```python
from build123d import *

# Parameters (mm, degrees)
BOSS_EXTRUDE1_DEPTH = 1
SKETCH2_W           = 7
SKETCH2_H           = 18
SKETCH2_R           = 2
BOSS_EXTRUDE2_DEPTH = 4


with BuildPart() as part:
    # Sketch1 → Boss-Extrude1 (new body)
    with BuildSketch(Plane(origin=(0, 0, 0), x_dir=(1, 0, 0), z_dir=(0, 1, 0))):
        Polygon((-9, 0), (9, 0), (9, 3), (6, 3), (6, 14), (9, 14), (9, 18), (-9, 18), (-9, 14), (-6, 14), (-6, 3), (-9, 3), align=None)
    extrude(amount=BOSS_EXTRUDE1_DEPTH)

    # Sketch2 → Boss-Extrude2 (add)
    # profile 1 of 2: a face of its own
    with BuildSketch(Plane(origin=(0, 1, 0), x_dir=(1, 0, 0), z_dir=(0, 1, 0))):
        with Locations((-12.5, 9)):
            Rectangle(SKETCH2_W, SKETCH2_H)
        with Locations(Location((-12.5, 9, 0), (0, 0, 270))):
            Circle(SKETCH2_R, mode=Mode.SUBTRACT)
    # profile 2 of 2: a face of its own
    with BuildSketch(Plane(origin=(0, 1, 0), x_dir=(1, 0, 0), z_dir=(0, 1, 0))):
        with Locations((12.5, 9)):
            Rectangle(SKETCH2_W, SKETCH2_H)
        with Locations(Location((12.5, 9, 0), (0, 0, 90))):
            Circle(SKETCH2_R, mode=Mode.SUBTRACT)
    extrude(amount=-BOSS_EXTRUDE2_DEPTH)


solid = part.part
```
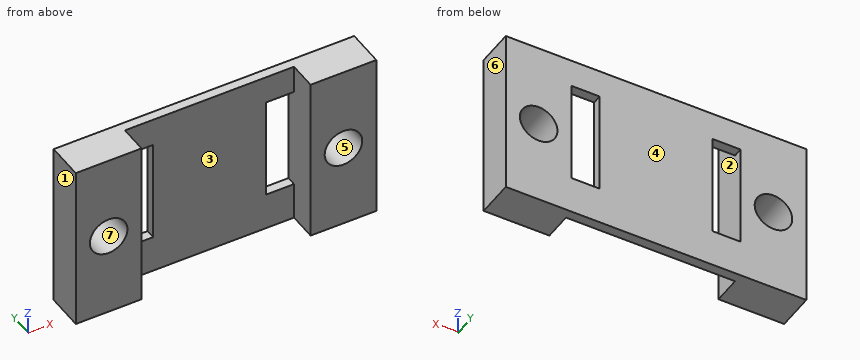
Check sheet for the modelled part. Datum: model origin and axes. Units: mm. Face numbers are marked on the shaded views. A direction names the side the tool comes from. Coordinates: 2 decimals unless noted, no trailing zeros. Write each loop counter-clockwise with the first axis right and the second up, starting at its lowest first coordinate (ties: lowest second). Pieces come first, ordered by that corner, then holes. Notation, with made-up numbers: (56.25, -26) - (66.25, -26) arc R21 ccw to (66.25, -1) - close; hole circle Ø7 at (22, 25). An arc over 180 degrees is marked (long way). One line per question, with ' | ' between items.
Item 1: Thickness scan on line 1 (X direction, y = -1.7, z = -9); line 2 (X direction, y = 0.5, z = -13.25); line 3 (Z direction, x = 12.5, y = -0.7). Record the ranges inside material, lowest first. Write a range as [from, to].
Determined:
line 1: x = [-16, -14.5], [-10.5, -9], [9, 10.5], [14.5, 16] | line 2: x = [-16, -9], [-6, 6], [9, 16] | line 3: z = [-18, -11], [-7, 0]
Item 2: Mould release check, pull along X, two halves, no side actions. Record for the marked faces 4, 5, 6 and 7: pulls with the +X half, pulls with the -X half, needs draft (parallel to the pull), parting line crosses it, or undercut.
Determined:
face 4: needs draft | face 5: undercut | face 6: pulls with the +X half | face 7: undercut
Item 3: Sectioned sample at A-A on y = -1.8. Record the boundary of the cut face in (x, z).
Determined:
outline: (-16, -18) - (-9, -18) - (-9, 0) - (-16, 0) - close; (9, -18) - (16, -18) - (16, 0) - (9, 0) - close; hole circle Ø4 at (-12.5, -9); hole circle Ø4 at (12.5, -9)
Item 4: Gauge pin test, flat ends, axial feed: P1, Ø1.5, axis at x = 3.5, y = -2.5, coming from the -Z side; P2, Ø2, axis at x = -3, z = -3.5, coming from the -Y side. Record the tip position at first contact, or that the pin passes through.
Determined:
P1: passes through | P2: stops at y = 0
Item 5: Access from +Z, -Z, +X, -X, +Y, -Y to the whole of each face (thin tool, end or side, straight path). Record for the marked faces 1, 2 and 3.
Determined:
face 1: +Z, -Z, -X, +Y, -Y | face 2: -Y | face 3: +Z, -Z, -Y
Item 6: Sectioned sample at C-C on z = -9. Record the boundary of the cut face in (x, y), plus the area to 3 significant figures.
Determined:
outline: (-16, -3) - (-14.5, -3) - (-14.5, 1) - (-16, 1) - close; (-10.5, -3) - (-9, -3) - (-9, 1) - (-10.5, 1) - close; (-6, 0) - (6, 0) - (6, 1) - (-6, 1) - close; (9, -3) - (10.5, -3) - (10.5, 1) - (9, 1) - close; (14.5, -3) - (16, -3) - (16, 1) - (14.5, 1) - close | area: 36.0 mm2
Item 7: Sectioned sample at B-B on x = -12.5. Record the boundary of the cut face in (y, z).
Determined:
outline: (-3, -18) - (1, -18) - (1, -11) - (-3, -11) - close; (-3, -7) - (1, -7) - (1, 0) - (-3, 0) - close
Item 8: Sectioned sample at D-D on y = 0.5. Record the boundary of the cut face in (x, z).
Determined:
outline: (-16, -18) - (16, -18) - (16, 0) - (-16, 0) - close; hole circle Ø4 at (-12.5, -9); hole (-9, -14) - (-6, -14) - (-6, -3) - (-9, -3) - close; hole (6, -14) - (9, -14) - (9, -3) - (6, -3) - close; hole circle Ø4 at (12.5, -9)
